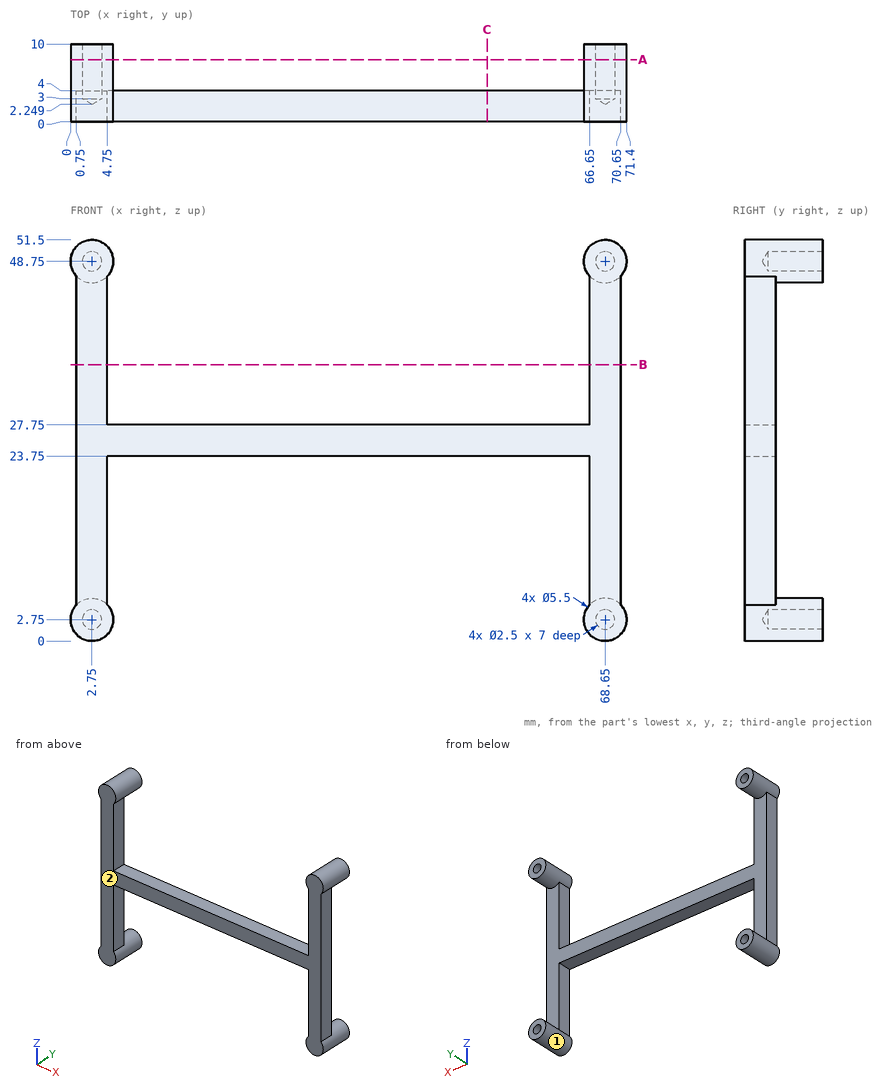
Can you work these out from the drawing? Everything is in mm from the part's minimum corner. Give positions to 0.01 mm unless a question says otherwise; leave off trailing zeros. Loops run counter-clockwise (first coordinate to the right, second up) from the corner with the lowest first, then second, coordinate; pieces in that order, holes last. Notation, with made-up numbers: (58.5, 6.5) -> (79.5, 6.5) arc R15 ccw to (79.5, 20.5) -> close; hole circle Ø8 at (67, -37). An arc over 180 degrees is marked (long way). Put each result on its own line as item: value.
(1) Thinking about a two-plate mould opening in Z: for the marked faces 1 and 2, which applies, pulls with the +Z half, pulls with the -Z half, needs draft (parallel to the pull), parting line crosses it, or undercut?
Computed:
face 1: undercut
face 2: needs draft
(2) Please list where these lines run through material, in increasing order: probe 1 along X at (y, z) = (6.5, 48.75); probe 2 along Z at (x, y) = (2.75, 8.25); probe 3 along X at (y, z) = (3, 46). Write a range as [from, to].
Computed:
probe 1: [0, 1.5], [4, 5.5], [65.9, 67.4], [69.9, 71.4]
probe 2: [0, 1.5], [4, 5.5], [46, 47.5], [50, 51.5]
probe 3: [0.75, 4.75], [66.65, 70.65]
(3) Imagine slicing it at B-B on z = 35.5. Write out the boundary of the cut face in (x, y), plus the area to 3 significant figures.
Computed:
outline: (0.75, 0) -> (4.75, 0) -> (4.75, 4) -> (0.75, 4) -> close; (66.65, 0) -> (70.65, 0) -> (70.65, 4) -> (66.65, 4) -> close
area: 32.0 mm^2
(4) I'm going to push flat-ended pins straight in: pin 1 Ø6 at (y, z) = (2.5, 34) entering from +X; pin 2 Ø6 at (x, y) = (55.5, 2.5) entering from -Z; pin 3 Ø4.5 at (y, z) = (1, 11) entering from -X. Where does each tip first touch, or does it pass through?
Computed:
pin 1: x = 70.65
pin 2: z = 23.75
pin 3: x = 0.75
(5) Imagine slicing it at C-C on x = 53.5. Write out the boundary of the cut face in (y, z).
Computed:
outline: (0, 23.75) -> (4, 23.75) -> (4, 27.75) -> (0, 27.75) -> close
(6) Imagine slicing it at A-A on y = 8. Write out the boundary of the cut face in (x, z).
Computed:
outline: circle Ø5.5 at (2.75, 2.75); circle Ø5.5 at (2.75, 48.75); circle Ø5.5 at (68.65, 2.75); circle Ø5.5 at (68.65, 48.75); hole circle Ø2.5 at (2.75, 2.75); hole circle Ø2.5 at (2.75, 48.75); hole circle Ø2.5 at (68.65, 2.75); hole circle Ø2.5 at (68.65, 48.75)
